Input: part model. Units: mm. Frame: model coordinates. Face numbers are marked on the shaded views. A direction names the side the tool comes from. Give positions to 0.01 mm unless a question says otherwise; leave off trailing zeros. Order: outer loops, then holes, each group sorted by start corner. A loop starts at its lowest first (then second) coordinate and runs counter-clockwise, first axis right, second up. Notation, with made-up numbers: (74.5, -34.75) - (99.5, -34.75) arc R18 ccw to (99.5, -12.75) - close; hole circle Ø6 at (78.25, 39.5). An arc over 180 degrees is marked (long way). Use a Markdown table: item, result.
from build123d import *

# Parameters (mm, degrees)
CROQUIS1_R              = 10
CROQUIS1_R_2            = 3.5
EXTRUIR1_DEPTH          = 12
CROQUIS2_W              = 45
CROQUIS2_H              = 22
SALIENTE_EXTRUIR1_DEPTH = 5
REDONDEO1_R             = 5
REDONDEO2_R             = 5
REDONDEO3_R             = 5
REDONDEO4_R             = 5
CROQUIS3_R              = 4.1
CORTAR_EXTRUIR1_DEPTH   = 45
CROQUIS4_R              = 1.55
CORTAR_EXTRUIR2_DEPTH   = 45
CROQUIS7_W              = 22.113905464
CROQUIS7_H              = 24
CORTAR_EXTRUIR4_DEPTH   = 70
CROQUIS8_W              = 45
CROQUIS8_H              = 22
SALIENTE_EXTRUIR2_DEPTH = 5
REDONDEO5_R             = 5
REDONDEO6_R             = 5
REDONDEO7_R             = 5
REDONDEO8_R             = 5
CORTAR_EXTRUIR5_START   = -15
CROQUIS9_R              = 1.55
CROQUIS9_R_2            = 4.1
CORTAR_EXTRUIR5_DEPTH   = 15
CROQUIS10_W             = 11.329180456
CROQUIS10_H             = 11.81266377
SALIENTE_EXTRUIR3_DEPTH = 10
CROQUIS11_W             = 64.145296703
CROQUIS11_H             = 8.366265536
CORTAR_EXTRUIR8_DEPTH   = 30
CROQUIS12_W             = 25
CROQUIS12_H             = 22
SALIENTE_EXTRUIR4_DEPTH = 70
CROQUIS13_W             = 19
CROQUIS13_H             = 16
CORTAR_EXTRUIR9_DEPTH   = 70
CROQUIS14_W             = 19
CROQUIS14_H             = 23
CORTAR_EXTRUIR10_DEPTH  = 70
CROQUIS15_W             = 16.823011057
CROQUIS15_H             = 23
CROQUIS15_W_2           = 14.386150498
CORTAR_EXTRUIR11_DEPTH  = 70
REDONDEO9_R             = 5
REDONDEO10_R            = 5
REDONDEO11_R            = 5
REDONDEO12_R            = 5
CROQUIS16_W             = 3
CROQUIS16_H             = 16
SALIENTE_EXTRUIR5_DEPTH = 47
CROQUIS17_W             = 22
CROQUIS17_H             = 23
SALIENTE_EXTRUIR6_DEPTH = 3
CROQUIS18_W             = 22
CROQUIS18_H             = 23
SALIENTE_EXTRUIR7_DEPTH = 3


with BuildPart() as part:
    # Croquis1 → Extruir1 (new body)
    with BuildSketch(Plane(origin=(0, 0, 0), x_dir=(1, 0, 0), z_dir=(0, 1, 0))):
        with Locations(Location((0, 0, 0), (0, 0, 270))):
            Circle(CROQUIS1_R)
        with Locations(Location((0, 0, 0), (0, 0, 270))):
            Circle(CROQUIS1_R_2, mode=Mode.SUBTRACT)
    extrude(amount=EXTRUIR1_DEPTH)

    # Croquis2 → Saliente-Extruir1 (add)
    with BuildSketch(Plane(origin=(0, 12, 0), x_dir=(1, 0, 0), z_dir=(0, 1, 0))):
        Rectangle(CROQUIS2_W, CROQUIS2_H)
    extrude(amount=SALIENTE_EXTRUIR1_DEPTH)

    # Redondeo1
    redondeo1_edges = [part.edges().sort_by_distance(p)[0] for p in [
        (22.5, 14.5, -11),
    ]]
    fillet(redondeo1_edges, radius=REDONDEO1_R)

    # Redondeo2
    redondeo2_edges = [part.edges().sort_by_distance(p)[0] for p in [
        (22.5, 14.5, 11),
    ]]
    fillet(redondeo2_edges, radius=REDONDEO2_R)

    # Redondeo3
    redondeo3_edges = [part.edges().sort_by_distance(p)[0] for p in [
        (-22.5, 14.5, 11),
    ]]
    fillet(redondeo3_edges, radius=REDONDEO3_R)

    # Redondeo4
    redondeo4_edges = [part.edges().sort_by_distance(p)[0] for p in [
        (-22.5, 14.5, -11),
    ]]
    fillet(redondeo4_edges, radius=REDONDEO4_R)

    # Croquis3 → Cortar-Extruir1 (cut)
    with BuildSketch(Plane.XZ):
        with Locations(Location((0, 0, 0), (0, 0, 270))):
            Circle(CROQUIS3_R)
    extrude(amount=-CORTAR_EXTRUIR1_DEPTH, mode=Mode.SUBTRACT)

    # Croquis4 → Cortar-Extruir2 (cut)
    with BuildSketch(Plane.XZ.offset(-12)):
        with Locations(Location((-16.5, 5, 0), (0, 0, 270))):
            Circle(CROQUIS4_R)
        with Locations(Location((-16.5, -5, 0), (0, 0, 270))):
            Circle(CROQUIS4_R)
        with Locations(Location((16.5, 5, 0), (0, 0, 270))):
            Circle(CROQUIS4_R)
        with Locations(Location((16.5, -5, 0), (0, 0, 270))):
            Circle(CROQUIS4_R)
    extrude(amount=-CORTAR_EXTRUIR2_DEPTH, mode=Mode.SUBTRACT)

    # Croquis7 → Cortar-Extruir4 (cut)
    with BuildSketch(Plane.XY.offset(11)):
        Rectangle(CROQUIS7_W, CROQUIS7_H)
    extrude(amount=-CORTAR_EXTRUIR4_DEPTH, mode=Mode.SUBTRACT)

    # Croquis8 → Saliente-Extruir2 (add)
    with BuildSketch(Plane.XZ.offset(-12)):
        Rectangle(CROQUIS8_W, CROQUIS8_H)
    extrude(amount=SALIENTE_EXTRUIR2_DEPTH)

    # Redondeo5
    redondeo5_edges = [part.edges().sort_by_distance(p)[0] for p in [
        (-22.5, 9.5, -11),
    ]]
    fillet(redondeo5_edges, radius=REDONDEO5_R)

    # Redondeo6
    redondeo6_edges = [part.edges().sort_by_distance(p)[0] for p in [
        (22.5, 9.5, -11),
    ]]
    fillet(redondeo6_edges, radius=REDONDEO6_R)

    # Redondeo7
    redondeo7_edges = [part.edges().sort_by_distance(p)[0] for p in [
        (22.5, 9.5, 11),
    ]]
    fillet(redondeo7_edges, radius=REDONDEO7_R)

    # Redondeo8
    redondeo8_edges = [part.edges().sort_by_distance(p)[0] for p in [
        (-22.5, 9.5, 11),
    ]]
    fillet(redondeo8_edges, radius=REDONDEO8_R)

    # Croquis9 → Cortar-Extruir5 (cut)
    with BuildSketch(Plane(origin=(0, 17, 0), x_dir=(1, 0, 0), z_dir=(0, 1, 0)).offset(CORTAR_EXTRUIR5_START)):
        with Locations(Location((-16.5, -5, 0), (0, 0, 90))):
            Circle(CROQUIS9_R)
        with Locations(Location((-16.5, 5, 0), (0, 0, 90))):
            Circle(CROQUIS9_R)
        with Locations(Location((16.5, -5, 0), (0, 0, 90))):
            Circle(CROQUIS9_R)
        with Locations(Location((16.5, 5, 0), (0, 0, 90))):
            Circle(CROQUIS9_R)
        with Locations(Location((0, 0, 0), (0, 0, 90))):
            Circle(CROQUIS9_R_2)
    extrude(amount=CORTAR_EXTRUIR5_DEPTH, mode=Mode.SUBTRACT)

    # Croquis10 → Saliente-Extruir3 (add)
    with BuildSketch(Plane(origin=(0, 17, 0), x_dir=(1, 0, 0), z_dir=(0, 1, 0))):
        Rectangle(CROQUIS10_W, CROQUIS10_H)
    extrude(amount=-SALIENTE_EXTRUIR3_DEPTH)

    # Croquis11 → Cortar-Extruir8 (cut)
    with BuildSketch(Plane(origin=(0, 0, -11), x_dir=(-1, 0, 0), z_dir=(0, 0, -1))):
        with Locations((-4.603378936, 7.816867232)):
            Rectangle(CROQUIS11_W, CROQUIS11_H)
    extrude(amount=-CORTAR_EXTRUIR8_DEPTH, mode=Mode.SUBTRACT)

    # Croquis12 → Saliente-Extruir4 (add)
    with BuildSketch(Plane.XZ.offset(-12)):
        Rectangle(CROQUIS12_W, CROQUIS12_H)
    extrude(amount=SALIENTE_EXTRUIR4_DEPTH)

    # Croquis13 → Cortar-Extruir9 (cut)
    with BuildSketch(Plane.XZ.offset(58)):
        Rectangle(CROQUIS13_W, CROQUIS13_H)
    extrude(amount=-CORTAR_EXTRUIR9_DEPTH, mode=Mode.SUBTRACT)

    # Croquis14 → Cortar-Extruir10 (cut)
    with BuildSketch(Plane.XY.offset(11)):
        with Locations((0, -46.5)):
            Rectangle(CROQUIS14_W, CROQUIS14_H)
    extrude(amount=-CORTAR_EXTRUIR10_DEPTH, mode=Mode.SUBTRACT)

    # Croquis15 → Cortar-Extruir11 (cut)
    with BuildSketch(Plane(origin=(12.5, 0, 0), x_dir=(0, 0, -1), z_dir=(1, 0, 0))):
        with Locations((-16.411505529, -46.5)):
            Rectangle(CROQUIS15_W, CROQUIS15_H)
        with Locations((15.193075249, -46.5)):
            Rectangle(CROQUIS15_W_2, CROQUIS15_H)
    extrude(amount=-CORTAR_EXTRUIR11_DEPTH, mode=Mode.SUBTRACT)

    # Redondeo9
    # the kernel refuses this fillet: 5 mm, written as the material it adds along each edge
    with BuildSketch(Plane(origin=(-9.5, -35, -8), x_dir=(0, 0, -1), z_dir=(-1, 0, 0))) as redondeo9_piece_1:
        with BuildLine():
            CenterArc((5, 4.582575695), REDONDEO9_R, 180, 66.421821522)
            Line((0, 4.582575695), (0, 0))
            Line((0, 0), (3, 0))
        make_face()
    extrude(amount=3)

    # Redondeo10
    # the kernel refuses this fillet: 5 mm, written as the material it adds along each edge
    with BuildSketch(Plane(origin=(12.5, -35, -8), x_dir=(0, 0, -1), z_dir=(-1, 0, 0))) as redondeo10_piece_1:
        with BuildLine():
            CenterArc((5, 4.582575695), REDONDEO10_R, 180, 66.421821522)
            Line((0, 4.582575695), (0, 0))
            Line((0, 0), (3, 0))
        make_face()
    extrude(amount=3)

    # Redondeo11
    # the kernel refuses this fillet: 5 mm, written as the material it adds along each edge
    with BuildSketch(Plane(origin=(-9.5, -35, 8), x_dir=(0, 0, 1), z_dir=(-1, 0, 0))) as redondeo11_piece_1:
        with BuildLine():
            CenterArc((5, -4.582575695), REDONDEO11_R, 113.578178478, 66.421821522)
            Line((0, -4.582575695), (0, 0))
            Line((0, 0), (3, 0))
        make_face()
    extrude(amount=3)

    # Redondeo12
    # the kernel refuses this fillet: 5 mm, written as the material it adds along each edge
    with BuildSketch(Plane(origin=(12.5, -35, 8), x_dir=(0, 0, 1), z_dir=(-1, 0, 0))) as redondeo12_piece_1:
        with BuildLine():
            CenterArc((5, -4.582575695), REDONDEO12_R, 113.578178478, 66.421821522)
            Line((0, -4.582575695), (0, 0))
            Line((0, 0), (3, 0))
        make_face()
    extrude(amount=3)

    # Croquis16 → Saliente-Extruir5 (add)
    with BuildSketch(Plane.XZ.offset(-12)):
        Rectangle(CROQUIS16_W, CROQUIS16_H)
    extrude(amount=SALIENTE_EXTRUIR5_DEPTH)

    # Croquis17 → Saliente-Extruir6 (add)
    with BuildSketch(Plane(origin=(12.5, 0, 0), x_dir=(0, 0, -1), z_dir=(1, 0, 0))):
        with Locations((0, -46.5)):
            Rectangle(CROQUIS17_W, CROQUIS17_H)
    extrude(amount=-SALIENTE_EXTRUIR6_DEPTH)

    # Croquis18 → Saliente-Extruir7 (add)
    with BuildSketch(Plane.ZY.offset(12.5)):
        with Locations((0, -46.5)):
            Rectangle(CROQUIS18_W, CROQUIS18_H)
    extrude(amount=-SALIENTE_EXTRUIR7_DEPTH)


solid = part.part
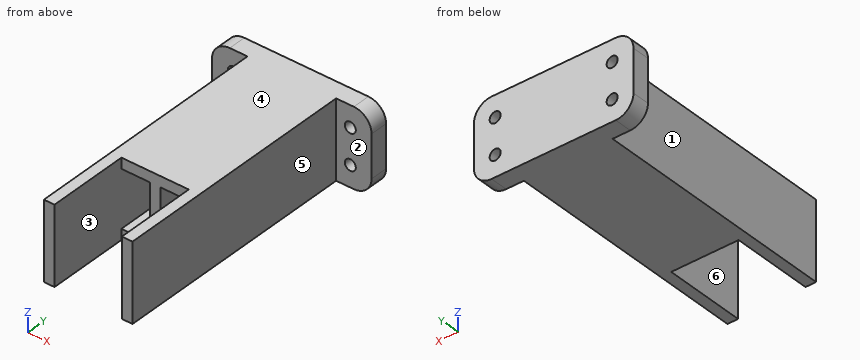
1. Section query B-B (y = -28). Return loops of the section in (x, z), then the cut area to 3 significant figures.
Response:
| item | result |
|---|---|
| outline | (-12.5, -11) - (12.5, -11) - (12.5, 11) - (-12.5, 11) - close; hole (-9.5, -8) - (-1.5, -8) - (-1.5, 8) - (-9.5, 8) - close; hole (1.5, -8) - (9.5, -8) - (9.5, 8) - (1.5, 8) - close |
| area | 294 mm^2 |
2. Section query D-D (z = -9). Return loops of the section in (x, y).
Response:
| item | result |
|---|---|
| outline | (-21.5, 12) - (-12.5, 12) - (-12.5, -58) - (-9.5, -58) - (-9.5, -35) - (9.5, -35) - (9.5, -58) - (12.5, -58) - (12.5, 12) - (21.5, 12) - (21.5, 17) - (-21.5, 17) - close |
3. Pin query (flat end, axial travel): pin 1 (8 mm diameter, centred on y = 4.5, z = -1, fed in from -X); pin 2 (6.5 mm diameter, centred on y = -35.5, z = -2.5, fed in from +X); pin 3 (2 mm diameter, centred on x = 14, z = -3, fed in from -Y). Return the tip coordinate at first contact, or that it passes through.
Response:
| item | result |
|---|---|
| pin 1 | stops at x = -12.5 |
| pin 2 | stops at x = 12.5 |
| pin 3 | stops at y = 12 |
4. Set-up query: the marked faces 1, 2 and 3. Return all of +Z, -Z, +X, -X, +Y, -Y with unobstructed straight access to the full face (end or side cutting, diameter ignored); none if empty.
Response:
| item | result |
|---|---|
| face 1 | +Z, -Z, -X, -Y |
| face 2 | +Z, -Z, +X, -Y |
| face 3 | -Y |
5. Mould query, pull axis Z, two halves, no side actions, for the marked faces 4, 5 and 6. Classes: pulls with the +Z half, pulls with the -Z half, needs draft (parallel to the pull), parting line crosses it, or undercut.
Response:
| item | result |
|---|---|
| face 4 | pulls with the +Z half |
| face 5 | needs draft |
| face 6 | undercut |
6. Material intervals for line 1 along X through (y, z) = (14, 5); line 2 along X through (y, z) = (-22, 2); line 3 along X through (y, z) = (-36, -1.25), sorted ascending.
Response:
| item | result |
|---|---|
| line 1 | x = -22.5 to -18.05, -14.95 to 14.95, 18.05 to 22.5 |
| line 2 | x = -12.5 to -9.5, -1.5 to 1.5, 9.5 to 12.5 |
| line 3 | x = -12.5 to -9.5, 9.5 to 12.5 |
7. Section query C-C (x = 16.5). Return loops of the section in (y, z).
Response:
| item | result |
|---|---|
| outline | (12, -11) - (17, -11) - (17, -6.55) - (12, -6.55) - close; (12, -3.45) - (17, -3.45) - (17, 3.45) - (12, 3.45) - close; (12, 6.55) - (17, 6.55) - (17, 11) - (12, 11) - close |
8. Section query A-A (z = -5). Return loops of the section in (x, y).
Response:
| item | result |
|---|---|
| outline | (-22.5, 12) - (-18.05, 12) - (-18.05, 17) - (-22.5, 17) - close; (-14.95, 12) - (-12.5, 12) - (-12.5, -58) - (-9.5, -58) - (-9.5, 12) - (-1.5, 12) - (-1.5, -35) - (1.5, -35) - (1.5, 12) - (9.5, 12) - (9.5, -58) - (12.5, -58) - (12.5, 12) - (14.95, 12) - (14.95, 17) - (-14.95, 17) - close; (18.05, 12) - (22.5, 12) - (22.5, 17) - (18.05, 17) - close |
